Geometry check sheet. Reference: the model listing, model coordinates, mm. Coordinates: 2 decimals unless noted, no trailing zeros. Loops run counter-clockwise (first coordinate to the right, second up) from the corner with the lowest first, then second, coordinate; pieces in that order, holes last.
from build123d import *

# Parameters (mm, degrees)
BOSS_EXTRUDE1_DEPTH  = 2.4
M3_CLEARANCE_HOLE1_D = 3.4
CIRPATTERN1_COUNT    = 6


with BuildPart() as part:
    # Sketch1 → Boss-Extrude1 (new body)
    with BuildSketch(Plane(origin=(0, 0, 0), x_dir=(1, 0, 0), z_dir=(0, 1, 0))):
        with BuildLine():
            ThreePointArc((-42.969094344, -11.378024049), (-44.45, 0), (-42.969094344, 11.378024049))
            ThreePointArc((-42.969094344, 11.378024049), (-46.651327743, 7.715429023), (-48, 2.7))
            Line((-48, 2.7), (-48, -2.7))
            ThreePointArc((-48, -2.7), (-46.651327743, -7.715429023), (-42.969094344, -11.378024049))
        make_face()
        with BuildLine():
            Line((38, 12.7), (-38, 12.7))
            ThreePointArc((-38, 12.7), (-40.570968641, 12.363856386), (-42.969094344, 11.378024049))
            ThreePointArc((-42.969094344, 11.378024049), (-44.45, 0), (-42.969094344, -11.378024049))
            ThreePointArc((-42.969094344, -11.378024049), (-40.570968641, -12.363856386), (-38, -12.7))
            Line((-38, -12.7), (38, -12.7))
            ThreePointArc((38, -12.7), (40.570968641, -12.363856386), (42.969094344, -11.378024049))
            ThreePointArc((42.969094344, -11.378024049), (44.078218791, -5.736996445), (44.45, 0))
            ThreePointArc((44.45, 0), (44.078218791, 5.736996445), (42.969094344, 11.378024049))
            ThreePointArc((42.969094344, 11.378024049), (40.570968641, 12.363856386), (38, 12.7))
        make_face()
        with BuildLine():
            ThreePointArc((-38, -12.7), (-40.570968641, -12.363856386), (-42.969094344, -11.378024049))
            ThreePointArc((-42.969094344, -11.378024049), (0, -44.45), (42.969094344, -11.378024049))
            ThreePointArc((42.969094344, -11.378024049), (40.570968641, -12.363856386), (38, -12.7))
            Line((38, -12.7), (-38, -12.7))
        make_face()
        with BuildLine():
            ThreePointArc((-42.969094344, 11.378024049), (-40.570968641, 12.363856386), (-38, 12.7))
            Line((-38, 12.7), (38, 12.7))
            ThreePointArc((38, 12.7), (40.570968641, 12.363856386), (42.969094344, 11.378024049))
            ThreePointArc((42.969094344, 11.378024049), (0, 44.45), (-42.969094344, 11.378024049))
        make_face()
        with BuildLine():
            ThreePointArc((48, 2.7), (46.651327743, 7.715429023), (42.969094344, 11.378024049))
            ThreePointArc((42.969094344, 11.378024049), (44.078218791, 5.736996445), (44.45, 0))
            ThreePointArc((44.45, 0), (44.078218791, -5.736996445), (42.969094344, -11.378024049))
            ThreePointArc((42.969094344, -11.378024049), (46.651327743, -7.715429023), (48, -2.7))
            Line((48, -2.7), (48, 2.7))
        make_face()
    extrude(amount=BOSS_EXTRUDE1_DEPTH)

    # M3 Clearance Hole1 (through all)
    with Locations(Plane(origin=(0, 2.4, -41.275), x_dir=(0, 0, 1), z_dir=(0, 1, 0))):
        with Locations((0, 0)):
            m3_clearance_hole1 = Hole(M3_CLEARANCE_HOLE1_D / 2)

    # CirPattern1: M3 Clearance Hole1 ×6 about axis
    cirpattern1_axis = Axis((0, 0, 0), (0, 1, 0))
    for i in range(1, CIRPATTERN1_COUNT):
        add(m3_clearance_hole1.rotate(cirpattern1_axis, i * 360 / CIRPATTERN1_COUNT), mode=Mode.SUBTRACT)


solid = part.part
1) Section check B-B on y = 1.8. Count the separate pieces of the cut face and the enclosed holes in it, and give its area (3 significant figures).
Data:
separate pieces: 1
enclosed holes: 6
area: 6,290 mm2
2) Section check C-C on x = 23.5. Record the cut outline in (y, z), and give its area (3 significant figures).
Data:
outline: (0, -37.73) - (2.4, -37.73) - (2.4, 37.73) - (0, 37.73) - close
area: 181 mm2
3) Section check A-A on x = 0. Record the cut outline in (y, z) (3 decimals), and give its area (3 significant figures).
Data:
outline: (0, -44.45) - (2.4, -44.45) - (2.4, -42.975) - (0, -42.975) - close; (0, -39.575) - (2.4, -39.575) - (2.4, 39.575) - (0, 39.575) - close; (0, 42.975) - (2.4, 42.975) - (2.4, 44.45) - (0, 44.45) - close
area: 197 mm2
4) Mould release check, pull along Z, two halves, no side actions. Record for faces 1 (the cylindrical face through (-0.816, 1.183, 44.443)), 2 (the cylindrical face through (34.312, 1.183, -19.724)), 3 (the cylindrical face through (-46.6, 1.2, -7.8)), 4 (the cylindrical face through (-34.312, 1.183, 19.724)): +Z half, -Z half, draft (parallel to the pull), parting line (faces both ways), or undercut.
Data:
face 1: +Z half
face 2: undercut
face 3: -Z half
face 4: undercut
5) Section check D-D on z = 33. Record the cut outline in (x, y), and give its area (3 significant figures).
Data:
outline: (-29.78, 0) - (29.78, 0) - (29.78, 2.4) - (-29.78, 2.4) - close
area: 143 mm2
6) Material ranges on probe 1 along Z at (x, y) = (-1, 0.35); probe 2 along X at (y, z) = (0.4, -21); probe 3 along X at (y, z) = (0.35, 19.5), recorded low to high.
Data:
probe 1: z = -44.44 to -42.65, -39.9 to 39.9, 42.65 to 44.44
probe 2: x = -39.18 to -37.41, -34.08 to 34.08, 37.41 to 39.18
probe 3: x = -39.94 to -37.01, -34.48 to 34.48, 37.01 to 39.94
7) Depth check by flat-ended pin: pin 1 (3 mm diameter, centred on x = 35.75, z = -20.64, fed in from +Y). Enter the tip coordinate at first touch or a pass-through.
Data:
pin 1: passes through
